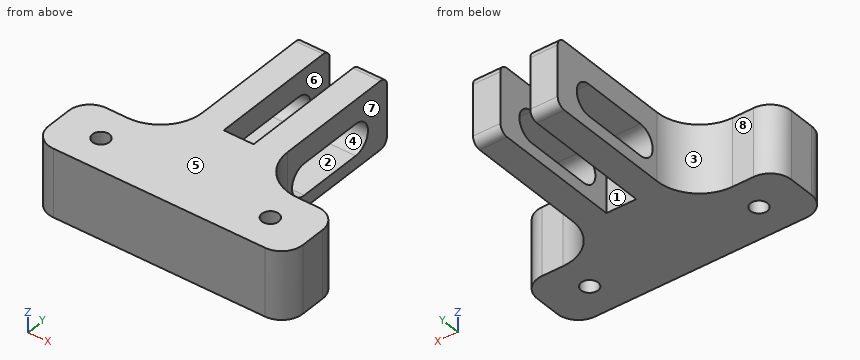
from build123d import *

# Parameters (mm, degrees)
SKETCH_W        = 60
SKETCH_H        = 16
SKETCH_R        = 2
PAD_DEPTH       = 16
SKETCH002_W     = 20
SKETCH002_H     = 16
PAD001_DEPTH    = 40
SKETCH003_W     = 7.05
SKETCH003_H     = 32
POCKET_DEPTH    = 16.001
POCKET001_DEPTH = 40.001
FILLET_R        = 10
FILLET001_R     = 2
FILLET002_R     = 5


with BuildPart() as part:
    # Sketch → Pad (new body)
    with BuildSketch(Plane.XY):
        with Locations((30, 8)):
            Rectangle(SKETCH_W, SKETCH_H)
        with Locations((10, 8)):
            Circle(SKETCH_R, mode=Mode.SUBTRACT)
        with Locations((50, 8)):
            Circle(SKETCH_R, mode=Mode.SUBTRACT)
    extrude(amount=PAD_DEPTH)

    # Sketch002 (on Face3 of Pad) → Pad001 (join)
    with BuildSketch(Plane(origin=(0, 16, 0), x_dir=(-1, 0, 0), z_dir=(0, 1, 0))):
        with Locations((-30, 8)):
            Rectangle(SKETCH002_W, SKETCH002_H)
    extrude(amount=PAD001_DEPTH)

    # Sketch003 (on Face12 of Pad001) → Pocket (cut, through all)
    with BuildSketch(Plane.XY.offset(16)):
        with Locations((30, 40)):
            Rectangle(SKETCH003_W, SKETCH003_H)
    extrude(amount=-POCKET_DEPTH, mode=Mode.SUBTRACT)

    # Sketch004 (on Face8 of Pocket) → Pocket001 (cut, through all)
    with BuildSketch(Plane.YZ.offset(40)):
        with BuildLine():
            ThreePointArc((31.02, 10.4), (27.32, 6.7), (31.02, 3))
            Line((31.02, 3), (46.55, 3))
            ThreePointArc((46.55, 3), (50.25, 6.7), (46.55, 10.4))
            Line((31.02, 10.4), (46.55, 10.4))
        make_face()
    extrude(amount=-POCKET001_DEPTH, mode=Mode.SUBTRACT)

    # Fillet
    fillet_edges = [part.edges().sort_by_distance(p)[0] for p in [
        (20, 16, 8),
        (40, 16, 8),
    ]]
    fillet(fillet_edges, radius=FILLET_R)

    # Fillet001
    fillet001_edges = [part.edges().sort_by_distance(p)[0] for p in [
        (36.7625, 56, 16),
        (23.2375, 56, 16),
        (23.2375, 56, 0),
        (36.7625, 56, 0),
    ]]
    fillet(fillet001_edges, radius=FILLET001_R)

    # Fillet002
    fillet002_edges = [part.edges().sort_by_distance(p)[0] for p in [
        (0, 16, 8),
        (0, 0, 8),
        (60, 0, 8),
        (60, 16, 8),
    ]]
    fillet(fillet002_edges, radius=FILLET002_R)


solid = part.part
Model file for the job. Use its own axes, mm. Face numbers are marked on the shaded views. A direction names the side the tool comes from. Coordinates: 2 decimals unless noted, no trailing zeros. Loops run counter-clockwise (first coordinate to the right, second up) from the corner with the lowest first, then second, coordinate; pieces in that order, holes last. Notation, with made-up numbers: (30.25, -36) -> (56.25, -36) arc R21 ccw to (56.25, 0) -> close; hole circle Ø5 at (17, 80.5). An arc over 180 degrees is marked (long way). Use one line per item in the form item = value. Start each with the question number.
(1) Probe probe 1 along Y at (x, z) = (50, 10); probe 2 along X at (y, z) = (49, 12.25) (3 decimals); probe 3 along Z at (x, y) = (36.5, 34). List the from-to ranges inside material, lowest first. Write a range as from..to.
(2) Flat gauge pins, fed straight in: pin 1 (8 mm diameter, centred on y = 43, z = 5.5, fed in from +X); pin 2 (5 mm diameter, centred on y = 45, z = 11.5, fed in from -X); pin 3 (8 mm diameter, centred on x = 31.5, z = 7, fed in from +Y); pin 4 (1.5 mm diameter, centred on x = 53, z = 12, fed in from +Y). Where does each tip first touch, or does it go through?
(3) Tool access for the marked faces 4, 5, 6, 7 and 8: list every direction of +Z, -Z, +X, -X, +Y, -Y with a clear straight run to the whole face (end or side of a thin tool).
(4) Cut at C-C on x = 39. Give the cut face in (y, z), and give its area (3 significant figures).
(5) Cut at B-B on y = 36.5. Give the cut face in (x, z) (3 decimals).
(6) Cut at D-D on y = 8. Give the cut face in (x, z).
(7) Pull direction X, two halves, no side cores. Call the marked faces 1, 2 and 3: pulls with the +X half, pulls with the -X half, needs draft (parallel to the pull), parting line crosses it, or undercut.
(8) Cut at A-A on z = 6.7. Give the cut face in (x, y) (3 decimals), and give its area (3 significant figures).
Values:
q1.probe_1 = 0..6, 10..16
q1.probe_2 = 20..26.475, 33.525..40
q1.probe_3 = 0..3, 10.4..16
q2.pin_1 = 40
q2.pin_2 = 20
q2.pin_3 = 56
q2.pin_4 = 16
q3.face_4 = +X, -X
q3.face_5 = +Z, +X, -X, +Y, -Y
q3.face_6 = +Z, -Z, +Y
q3.face_7 = +Z, -Z, +X, +Y
q3.face_8 = +Z, -Z, -X, +Y
q4.outline = (0, 0) -> (54, 0) arc R2 ccw to (56, 2) -> (56, 14) arc R2 ccw to (54, 16) -> (0, 16) -> close; hole (31.02, 3) -> (46.55, 3) arc R3.7 ccw to (46.55, 10.4) -> (31.02, 10.4) arc R3.7 ccw to start
q4.area = 736 mm2
q5.outline = (20, 0) -> (26.475, 0) -> (26.475, 3) -> (20, 3) -> close; (20, 10.4) -> (26.475, 10.4) -> (26.475, 16) -> (20, 16) -> close; (33.525, 0) -> (40, 0) -> (40, 3) -> (33.525, 3) -> close; (33.525, 10.4) -> (40, 10.4) -> (40, 16) -> (33.525, 16) -> close
q6.outline = (0, 0) -> (8, 0) -> (8, 16) -> (0, 16) -> close; (12, 0) -> (48, 0) -> (48, 16) -> (12, 16) -> close; (52, 0) -> (60, 0) -> (60, 16) -> (52, 16) -> close
q7.face_1 = undercut
q7.face_2 = needs draft
q7.face_3 = pulls with the -X half
q8.outline = (0, 5) arc R5 ccw to (5, 0) -> (55, 0) arc R5 ccw to (60, 5) -> (60, 11) arc R5 ccw to (55, 16) -> (50, 16) arc R10 cw to (40, 26) -> (40, 27.32) -> (33.525, 27.32) -> (33.525, 24) -> (26.475, 24) -> (26.475, 27.32) -> (20, 27.32) -> (20, 26) arc R10 cw to (10, 16) -> (5, 16) arc R5 ccw to (0, 11) -> close; (20, 50.25) -> (26.475, 50.25) -> (26.475, 56) -> (20, 56) -> close; (33.525, 50.25) -> (40, 50.25) -> (40, 56) -> (33.525, 56) -> close; hole circle Ø4 at (10, 8); hole circle Ø4 at (50, 8)
q8.area = 1,230 mm2
